```python
from build123d import *
from OCP.BRepFilletAPI import BRepFilletAPI_MakeFillet

# Parameters (mm, degrees)
SKETCH_1_R      = 1.35
EXTRUDE_1_DEPTH = 2
SKETCH_2_R      = 1.1
EXTRUDE_2_DEPTH = 2
FILLET_3_R1     = 3
FILLET_3_R2     = 4
FILLET_3_R3     = 2
FILLET_3_R4     = 8
FILLET_4_R      = 2


with BuildPart() as part:
    # 草图1 → 凸台-拉伸1 (new body)
    with BuildSketch(Plane(origin=(0, 0, 0), x_dir=(1, 0, 0), z_dir=(0, 1, 0))):
        Polygon((-13.5, -5), (13.5, -5), (13.5, 5), (-13.5, 5), (-23.5, 5), (-23.5, -5), align=None)
        with Locations(Location((7, 0, 0), (0, 0, 270))):
            Circle(SKETCH_1_R, mode=Mode.SUBTRACT)
        with Locations(Location((-9, 0, 0), (0, 0, 90))):
            Circle(SKETCH_1_R, mode=Mode.SUBTRACT)
        with Locations(Location((-18.5, 0, 0), (0, 0, 270))):
            Circle(SKETCH_1_R, mode=Mode.SUBTRACT)
    extrude(amount=EXTRUDE_1_DEPTH)

    # 草图2 → 凸台-拉伸2 (add)
    with BuildSketch(Plane(origin=(0, 2, 0), x_dir=(1, 0, 0), z_dir=(0, 1, 0))):
        with BuildLine():
            Line((13.5, -5), (13.5, -13))
            ThreePointArc((13.5, -13), (21.845175456, -25.956218669), (18.5, -41))
            Line((18.5, -41), (6.5, -41))
            Line((6.5, -41), (6.5, -33))
            Line((6.5, -33), (16.5, -33))
            ThreePointArc((16.5, -33), (15.184290219, -22.40785489), (7.5, -15))
            Line((7.5, -15), (7.5, -5))
            Line((7.5, -5), (13.5, -5))
        make_face()
        with Locations(Location((10, -39, 0), (0, 0, 270))):
            Circle(SKETCH_2_R, mode=Mode.SUBTRACT)
        with Locations(Location((10, -35, 0), (0, 0, 90))):
            Circle(SKETCH_2_R, mode=Mode.SUBTRACT)
    extrude(amount=-EXTRUDE_2_DEPTH)

    # 圆角3: one fillet with a radius per group of edges: ONE call of the kernel's fillet builder (fillet() takes one radius for all edges)
    fillet_3_edges_1 = [part.edges().sort_by_distance(p)[0] for p in [
        (7.5, 1, 15),
    ]]
    fillet_3_edges_2 = [part.edges().sort_by_distance(p)[0] for p in [
        (13.5, 1, 13),
    ]]
    fillet_3_edges_3 = [part.edges().sort_by_distance(p)[0] for p in [
        (16.5, 1, 33),
    ]]
    fillet_3_edges_4 = [part.edges().sort_by_distance(p)[0] for p in [
        (18.5, 1, 41),
    ]]
    fillet_3 = BRepFilletAPI_MakeFillet(part.part.solid().wrapped)
    for e in fillet_3_edges_1:
        fillet_3.Add(FILLET_3_R1, e.wrapped)
    for e in fillet_3_edges_2:
        fillet_3.Add(FILLET_3_R2, e.wrapped)
    for e in fillet_3_edges_3:
        fillet_3.Add(FILLET_3_R3, e.wrapped)
    for e in fillet_3_edges_4:
        fillet_3.Add(FILLET_3_R4, e.wrapped)
    add(Compound.cast(fillet_3.Shape()), mode=Mode.REPLACE)

    # 圆角4
    fillet_4_edges = [part.edges().sort_by_distance(p)[0] for p in [
        (-23.5, 1, 5),
        (-23.5, 1, -5),
        (13.5, 1, -5),
        (7.5, 1, 5),
        (6.5, 1, 41),
        (6.5, 1, 33),
    ]]
    fillet(fillet_4_edges, radius=FILLET_4_R)


solid = part.part
```
Geometry: final body of the model. Coordinates: model frame, mm. A direction names the side the tool comes from. Round coordinates to 2 decimals unless told otherwise and drop trailing zeros. Write each loop counter-clockwise with the first axis right and the second up, starting at its lowest first coordinate (ties: lowest second). Pieces come first, ordered by that corner, then holes.
Item 1: Section query C-C (y = 1.3). Return loops of the section in (x, z), plus the area to 3 significant figures.
Item 2: Set-up query: faces 1 (the face through (13.5, 1, 4)), 2 (the face through (6.5, 1, 37)), 3 (the face through (6.9, 0.99, 5.57)). Return all of +Z, -Z, +X, -X, +Y, -Y with unobstructed straight access to the full face (end or side cutting, diameter ignored); none if empty.
Item 3: Section query B-B (x = -9). Return loops of the section in (y, z).
Item 4: Section query A-A (z = 0). Return loops of the section in (x, y), plus the area to 3 significant figures.
Item 5: Section query D-D (x = 10). Return loops of the section in (y, z).
Item 6: Mould query, pull axis X, two halves, no side actions, for faces 4 (the face through (12.93, 1.01, -4.4)), 5 (the face through (-19.7, 0.99, 0.62)), 6 (the face through (8.339, 0.986, -0.176)), 7 (the face through (-5, 1, -5)). Classes: +X half, -X half, draft (parallel to the pull), parting line (faces both ways), or undercut.
Item 7: Pin query (flat end, axial travel): P1, Ø1, axis at y = 1, z = 9, coming from the -X side; P2, Ø0.6, axis at x = -11.5, y = 0.5, coming from the +Z side; P3, Ø0.6, axis at y = 1, z = 38, coming from the -X side. Return the tip coordinate at first contact, or that it passes through.
Item 8: Material intervals for L1, parallel to X at y = 0.5, z = 0; L2, parallel to X at y = 1.6, z = 39; L3, parallel to X at y = 1.65, z = 29, sorted ascending.
Completed:
1. outline: (-23.5, -3) arc R2 ccw to (-21.5, -5) - (11.5, -5) arc R2 ccw to (13.5, -3) - (13.5, 11.02) arc R4 cw to (14.94, 14.09) arc R20 ccw to (21.27, 35.35) arc R8 ccw to (13.63, 41) - (8.5, 41) arc R2 ccw to (6.5, 39) - (6.5, 35) arc R2 ccw to (8.5, 33) - (14.8, 33) arc R2 cw to (16.79, 31.21) arc R16 cw to (8.98, 15.77) arc R3 ccw to (7.5, 13.18) - (7.5, 7) arc R2 cw to (5.5, 5) - (-21.5, 5) arc R2 ccw to (-23.5, 3) - close; hole circle Ø2.7 at (-18.5, 0); hole circle Ø2.7 at (-9, 0); hole circle Ø2.7 at (7, 0); hole circle Ø2.2 at (10, 35); hole circle Ø2.2 at (10, 39)
1. area: 618 mm2
2. face 1: -Z, +X, +Y, -Y
2. face 2: +Z, -X, +Y, -Y
2. face 3: -X, +Y, -Y
3. outline: (0, -5) - (2, -5) - (2, -1.35) - (0, -1.35) - close; (0, 1.35) - (2, 1.35) - (2, 5) - (0, 5) - close
4. outline: (-23.5, 0) - (-19.85, 0) - (-19.85, 2) - (-23.5, 2) - close; (-17.15, 0) - (-10.35, 0) - (-10.35, 2) - (-17.15, 2) - close; (-7.65, 0) - (5.65, 0) - (5.65, 2) - (-7.65, 2) - close; (8.35, 0) - (13.5, 0) - (13.5, 2) - (8.35, 2) - close
4. area: 57.8 mm2
5. outline: (0, -5) - (2, -5) - (2, 16.42) - (0, 16.42) - close; (0, 33) - (2, 33) - (2, 33.9) - (0, 33.9) - close; (0, 36.1) - (2, 36.1) - (2, 37.9) - (0, 37.9) - close; (0, 40.1) - (2, 40.1) - (2, 41) - (0, 41) - close
6. face 4: +X half
6. face 5: undercut
6. face 6: undercut
6. face 7: draft
7. P1: stops at x = 7.5
7. P2: stops at z = 5
7. P3: stops at x = 6.5
8. L1: x = -23.5 to -19.85, -17.15 to -10.35, -7.65 to 5.65, 8.35 to 13.5
8. L2: x = 6.5 to 8.9, 11.1 to 18.92
8. L3: x = 16.86 to 22.15
